```python
from build123d import *

# Parameters (mm, degrees)
F0_W     = 76.2
F0_H     = 76.2
F1_DEPTH = 76.2
F3_D     = 25.4
F4_W     = 25.4
F4_H     = 25.4
F5_DEPTH = 12.7
F6_R     = 12.7
F7_DEPTH = 12.7
F9_DEPTH = 25.4


with BuildPart() as f1:
    # F0 (on Front) → F1 (new body)
    with BuildSketch(Plane.XZ):
        with Locations((38.1, 114.3)):
            Rectangle(F0_W, F0_H)
    extrude(amount=F1_DEPTH)

    # F3 (through all)
    with Locations(Plane.XY.offset(152.4)):
        with Locations((38.483977, -38.1)):
            Hole(F3_D / 2)

    # F4 (on face) → F5 (join)
    with BuildSketch(Plane.XZ.offset(76.2)):
        with Locations((31.623321, 124.629789)):
            Rectangle(F4_W, F4_H)
    extrude(amount=F5_DEPTH)

    # F6 (on face) → F7 (join)
    with BuildSketch(Plane.YZ.offset(76.2)):
        with Locations((-26.029168, 105.892979)):
            Circle(F6_R)
    extrude(amount=F7_DEPTH)

    # F8 (on face) → F9 (join)
    with BuildSketch(Plane(origin=(0, 0, 0), x_dir=(-1, 0, 0), z_dir=(0, 1, 0))):
        Polygon((-28.910244, 106.993121), (-28.910244, 118.067446), (-38.50089, 123.604608), (-48.091536, 118.067446), (-48.091536, 106.993121), (-38.50089, 101.455959), align=None)
    extrude(amount=F9_DEPTH)


solid = f1.part
```
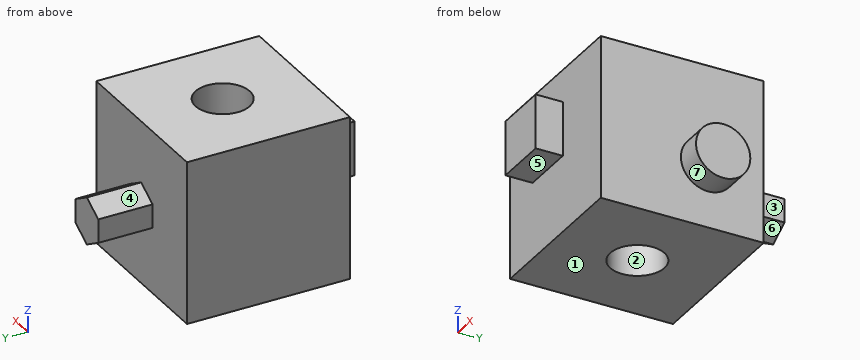
CAD build for the part. Positions are in the model's coordinates, mm. Face numbers are marked on the shaded views. A direction names the side the tool comes from. Give positions to 0.01 mm unless a question says otherwise; leave off trailing zeros. Order: outer loops, then holes, each group sorted by start corner. A loop starts at its lowest first (then second) coordinate and runs counter-clockwise, first axis right, second up. Notation, with made-up numbers: M 2.5,86 L 35.5,86 A13 ccw 35.5,102 Z; hole C 7,-7.5 d6. An arc over 180 degrees is marked long. Put each result on its own line as item: value. Start each with the question number.
(1) Saw through at B-B, the plane z = 100. Write the cut outline in (x, y), then the cut area to 3 significant figures.
(2) Saw through at A-A, the plane y = -43.5. Write the cut outline in (x, z), then the cut area to 3 significant figures.
(3) Which spindle directions (+Z, -Z, +X, -X, +Y, -Y) get a long thin tool onto all of the face, cutting with end or side? Do the marked faces 4, 5, 6 and 7. Say none if no direction does.
(4) Drill centre lines: line 1 along X through (y, z) = (-38, 95); line 2 along X through (y, z) = (-55, 97.5); line 3 along Y through (x, z) = (73.5, 84). Where is each one in solid material? Low to high.
(5) Mould opens along X. For the marked faces 1, 2 and 3 say: +X half, -X half, draft (parallel to the pull), parting line (faces both ways), or undercut.
(6) Saw through at C-C, the plane y = 8. Write the cut outline in (x, z).
(7) Flat gauge pins, fed straight in: pin 1 Ø14 at (x, y) = (37, -85.5) entering from +Z; pin 2 Ø4 at (y, z) = (-16.5, 95) entering from -X; pin 3 Ø3.5 at (y, z) = (16, 110.5) entering from +X; pin 4 Ø1.5 at (x, z) = (67, 144.5) entering from -Y. Where does each tip first touch, or does it go through?
(8) Saw through at D-D, the plane x = 73.5. Write the cut outline in (y, z).
Check result:
1. outline: M 0,-76.2 L 76.2,-76.2 L 76.2,-37.28 L 88.9,-37.28 L 88.9,-14.78 L 76.2,-14.78 L 76.2,0 L 0,0 Z; hole C 38.48,-38.1 d25.4
1. area: 5,590 mm2
2. outline: M 0,76.2 L 26.99,76.2 L 26.99,152.4 L 0,152.4 Z; M 49.98,76.2 L 76.2,76.2 L 76.2,152.4 L 49.98,152.4 Z
2. area: 4,050 mm2
3. face 4: +Z, -X, +Y
3. face 5: -Z, +X, -X, -Y
3. face 6: -Z, +X, +Y
3. face 7: +X
4. line 1: x = 0 to 25.78, 51.18 to 76.2
4. line 2: x = 0 to 76.2
4. line 3: y = -76.2 to 0
5. face 1: draft
5. face 2: undercut
5. face 3: +X half
6. outline: M 28.91,106.99 L 38.5,101.46 L 48.09,106.99 L 48.09,118.07 L 38.5,123.6 L 28.91,118.07 Z
7. pin 1: stops at z = 137.33
7. pin 2: stops at x = 0
7. pin 3: stops at x = 48.09
7. pin 4: stops at y = -76.2
8. outline: M -76.2,76.2 L 0,76.2 L 0,152.4 L -76.2,152.4 Z
